Design review of the part shown in the three views and the two pictorial views. Dimensions are in mm from the part's minimum x, y and z. Give positions to 0.01 mm unless a question says otherwise; leave off trailing zeros. Order: outer loops, then holes, each group sorted by start corner. A loop starts at its lowest first (then second) coordinate and runs counter-clockwise, first axis right, second up.
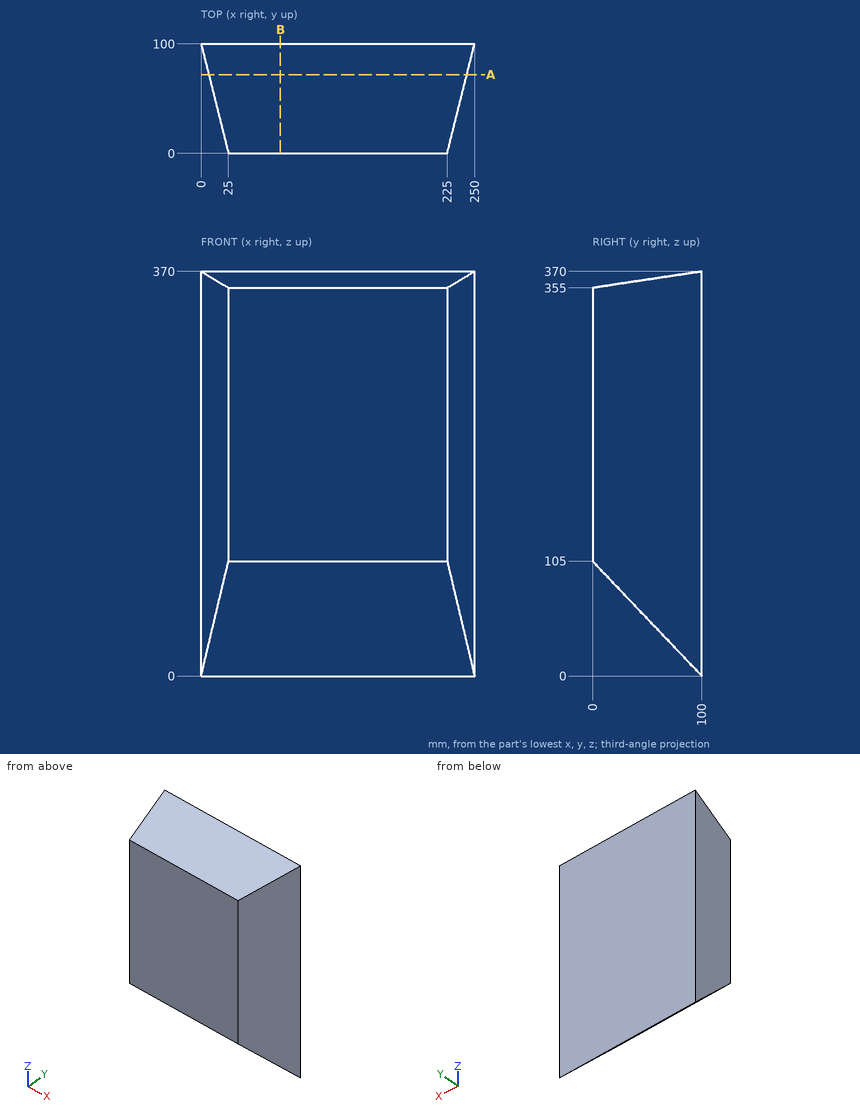
1) Clearance check with flat-ended pins moving along their axes: pin 1 (5 mm diameter, centred on y = 57.5, z = 311.5, fed in from +X); pin 2 (2 mm diameter, centred on x = 26.5, z = 45.5, fed in from -Y); pin 3 (8 mm diameter, centred on y = 69, z = 178, fed in from +X). State where each tip first meets the part, or that it passes through.
Answer sheet:
pin 1: stops at x = 240
pin 2: stops at y = 55.71
pin 3: stops at x = 243.25
2) To check wall thickness, follow line 1 (Y direction, x = 186, z = 41); line 2 (X direction, y = 89.5, z = 119) (3 decimals); line 3 (Y direction, x = 87.5, z = 66). State the ranges of each line that lie inside material, in increasing order.
Answer sheet:
line 1: y = 60.95 to 100
line 2: x = 2.625 to 247.375
line 3: y = 37.14 to 100
3) We need section B-B on x = 72.5. Give the boundary of the cut face in (y, z), then the cut area to 3 significant figures.
Answer sheet:
outline: (0, 105) - (100, 0) - (100, 370) - (0, 355) - close
area: 31,000 mm2
4) We need section A-A on y = 72. Give the boundary of the cut face in (x, z), then the cut area to 3 significant figures.
Answer sheet:
outline: (7, 29.4) - (243, 29.4) - (243, 365.8) - (7, 365.8) - close
area: 79,400 mm2
